Geometry: see drawing. Coordinates: mm, zero at the bounding-box minimum. Round coordinates to 2 decimals unless told otherwise and drop trailing zeros. Loops run counter-clockwise (first coordinate to the right, second up) from the corner with the lowest first, then second, coordinate; pieces in that order, holes last. Notation, with made-up numbers: (28.5, 84) -> (75.5, 84) arc R23 ccw to (75.5, 123) -> close; hole circle Ø10 at (-25, 74). An arc over 180 degrees is marked (long way). Write item = value, one per line.
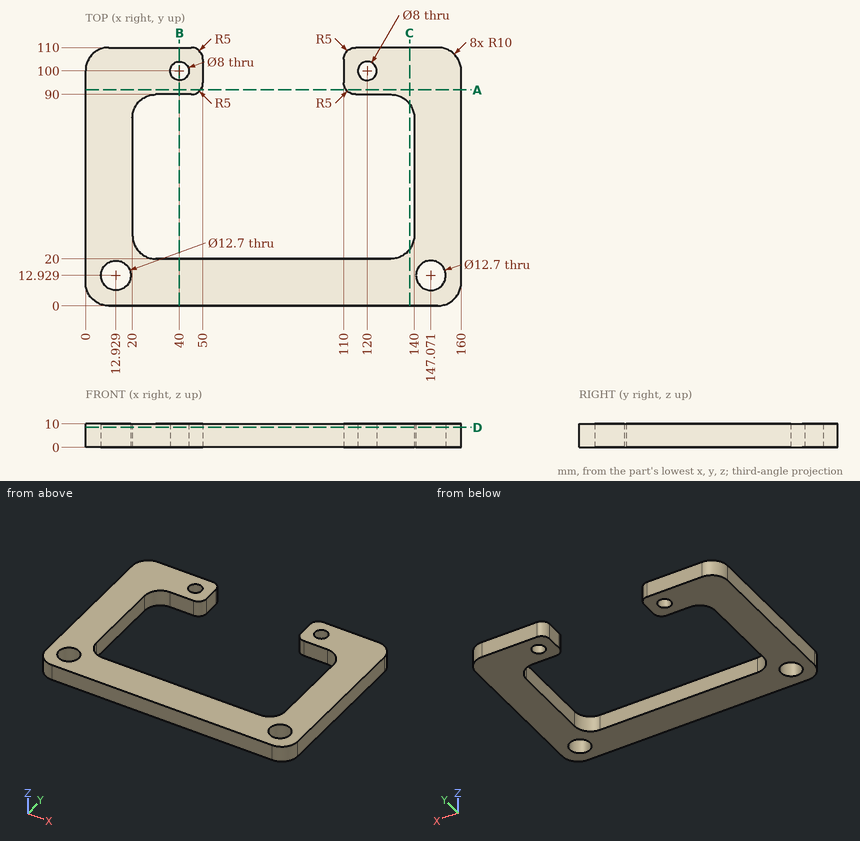
1. Section query C-C (x = 138). Return the cut outline in (y, z).
Evaluation:
outline = (0, 0) -> (24, 0) -> (24, 10) -> (0, 10) -> close; (86, 0) -> (110, 0) -> (110, 10) -> (86, 10) -> close
2. Section query B-B (x = 40). Return the cut outline in (y, z), then the cut area to 3 significant figures.
Evaluation:
outline = (0, 0) -> (20, 0) -> (20, 10) -> (0, 10) -> close; (90, 0) -> (96, 0) -> (96, 10) -> (90, 10) -> close; (104, 0) -> (110, 0) -> (110, 10) -> (104, 10) -> close
area = 320 mm²
3. Section query A-A (y = 92). Return the cut outline in (x, z), then the cut area to 3 significant figures.
Evaluation:
outline = (0, 0) -> (49, 0) -> (49, 10) -> (0, 10) -> close; (111, 0) -> (160, 0) -> (160, 10) -> (111, 10) -> close
area = 980 mm²
4. Section query D-D (z = 8.5). Return the cut outline in (x, y).
Evaluation:
outline = (0, 10) arc R10 ccw to (10, 0) -> (150, 0) arc R10 ccw to (160, 10) -> (160, 100) arc R10 ccw to (150, 110) -> (115, 110) arc R5 ccw to (110, 105) -> (110, 95) arc R5 ccw to (115, 90) -> (130, 90) arc R10 cw to (140, 80) -> (140, 30) arc R10 cw to (130, 20) -> (30, 20) arc R10 cw to (20, 30) -> (20, 80) arc R10 cw to (30, 90) -> (45, 90) arc R5 ccw to (50, 95) -> (50, 105) arc R5 ccw to (45, 110) -> (10, 110) arc R10 ccw to (0, 100) -> close; hole circle Ø12.7 at (12.93, 12.93); hole circle Ø8 at (40, 100); hole circle Ø8 at (120, 100); hole circle Ø12.7 at (147.07, 12.93)
5. Line query: probe 1 along X at (y, z) = (13, 8.25); probe 2 along X at (y, z) = (47, 5.5); probe 3 along X at (y, z) = (9.5, 5). Output: solid intervals per line, ascending. Write a range as from..to.
Evaluation:
probe_1 = 0..6.58, 19.28..140.72, 153.42..160
probe_2 = 0..20, 140..160
probe_3 = 0.01..7.58, 18.27..141.73, 152.42..159.99
6. Contact query for flat-ended pins moving along their axis: pin 1 Ø6 at (x, z) = (61.5, 8.5) entering from +Y; pin 2 Ø4 at (x, z) = (108.5, 5.5) entering from +Y. Output: stop coordinate, or through.
Evaluation:
pin_1 = 20
pin_2 = 107.18
